Can you work these out from the model? Positions are in its coordinate system, mm. A direction names the side the tool comes from. Coordinates: 2 decimals unless noted, no trailing zeros. Order: outer loops, then holes, each group sorted by start corner. A loop starts at its lowest first (then second) coordinate and runs counter-clockwise, first axis right, second up. Notation, with made-up numbers: (69.5, 7) -> (80.5, 7) arc R21 cw to (80.5, 16) -> close; hole circle Ø11 at (-26, 87.25). An arc over 180 degrees is marked (long way). Write item = value, one per line.
```python
from build123d import *

# Parameters (mm, degrees)
F0_W     = 19.506821
F0_H     = 90
F1_DEPTH = 9


with BuildPart() as f1:
    # F0 (on Front) → F1 (new body)
    with BuildSketch(Plane.XZ):
        with BuildLine():
            Line((100.506821, -115.94898), (100.506821, -102.44898))
            Line((100.506821, -102.44898), (81, -102.44898))
            Line((81, -102.44898), (81, -112.44898))
            ThreePointArc((81, -112.44898), (79.535534, -115.984513), (76, -117.44898))
            Line((76, -117.44898), (-76, -117.44898))
            ThreePointArc((-76, -117.44898), (-79.535534, -115.984513), (-81, -112.44898))
            Line((-81, -112.44898), (-81, -102.44898))
            Line((-81, -102.44898), (-101, -102.44898))
            Line((-101, -102.44898), (-101, -115.94898))
            ThreePointArc((-101, -115.94898), (-99.93934, -116.388319), (-99.5, -117.44898))
            ThreePointArc((-99.5, -117.44898), (-101, -118.94898), (-102.5, -117.44898))
            Line((-102.5, -117.44898), (-110, -117.44898))
            Line((-110, -117.44898), (-110, -122.44898))
            ThreePointArc((-110, -122.44898), (-104.142136, -136.591115), (-90, -142.44898))
            Line((-90, -142.44898), (90, -142.44898))
            ThreePointArc((90, -142.44898), (104.142136, -136.591115), (110, -122.44898))
            Line((110, -122.44898), (110, -117.44898))
            Line((110, -117.44898), (102.006821, -117.44898))
            ThreePointArc((102.006821, -117.44898), (99.446161, -118.50964), (100.506821, -115.94898))
        make_face()
        with Locations((90.753411, -57.44898)):
            Rectangle(F0_W, F0_H)
        with BuildLine():
            Line((90, 137.55102), (-90, 137.55102))
            ThreePointArc((-90, 137.55102), (-104.142136, 131.693156), (-110, 117.55102))
            Line((-110, 117.55102), (-110, 112.55102))
            Line((-110, 112.55102), (-102.5, 112.55102))
            ThreePointArc((-102.5, 112.55102), (-101, 114.05102), (-99.5, 112.55102))
            ThreePointArc((-99.5, 112.55102), (-99.93934, 111.49036), (-101, 111.05102))
            Line((-101, 111.05102), (-101, -12.44898))
            Line((-101, -12.44898), (-81, -12.44898))
            Line((-81, -12.44898), (-81, -7.44898))
            ThreePointArc((-81, -7.44898), (-79.535534, -3.913446), (-76, -2.44898))
            Line((-76, -2.44898), (-61, -2.44898))
            Line((-61, -2.44898), (-61, 17.55102))
            Line((-61, 17.55102), (-76, 17.55102))
            ThreePointArc((-76, 17.55102), (-79.535534, 19.015487), (-81, 22.55102))
            Line((-81, 22.55102), (-81, 107.55102))
            ThreePointArc((-81, 107.55102), (-79.535534, 111.086554), (-76, 112.55102))
            Line((-76, 112.55102), (76, 112.55102))
            ThreePointArc((76, 112.55102), (79.535534, 111.086554), (81, 107.55102))
            Line((81, 107.55102), (81, 22.55102))
            ThreePointArc((81, 22.55102), (79.535534, 19.015487), (76, 17.55102))
            Line((76, 17.55102), (60.506821, 17.55102))
            Line((60.506821, 17.55102), (60.506821, -2.44898))
            Line((60.506821, -2.44898), (76, -2.44898))
            ThreePointArc((76, -2.44898), (79.535534, -3.913446), (81, -7.44898))
            Line((81, -7.44898), (81, -12.44898))
            Line((81, -12.44898), (100.506821, -12.44898))
            Line((100.506821, -12.44898), (100.506821, 111.05102))
            ThreePointArc((100.506821, 111.05102), (99.446161, 113.611681), (102.006821, 112.55102))
            Line((102.006821, 112.55102), (110, 112.55102))
            Line((110, 112.55102), (110, 117.55102))
            ThreePointArc((110, 117.55102), (104.142136, 131.693156), (90, 137.55102))
        make_face()
    extrude(amount=-F1_DEPTH)


solid = f1.part
```
Item 1: If I drill on probe 1 along Z at (x, y) = (-64, 0.75); probe 2 along Z at (x, y) = (33, 7.5); probe 3 along X at (y, z) = (7.25, 2.5), over which ranges is the centre line in solid material (lowest first)?
A:
probe_1 = -142.45 to -117.45, -2.45 to 17.55, 112.55 to 137.55
probe_2 = -142.45 to -117.45, 112.55 to 137.55
probe_3 = -101 to -61, 60.51 to 100.51
Item 2: I want a section at A-A, the plane z = 88.5. Please give me the cut outline in (x, y), plus the area to 3 significant figures.
A:
outline = (-101, 0) -> (-81, 0) -> (-81, 9) -> (-101, 9) -> close; (81, 0) -> (100.51, 0) -> (100.51, 9) -> (81, 9) -> close
area = 356 mm2
Item 3: For faces 4 (the flat face through (-101, 4, 50)), 5 (the flat face through (106, 4, -117.449)), 6 (the cylindrical face through (104.297, 4.437, 131.537)), 7 (the flat face through (1, 4, 137.551)), 8 (the flat face through (-61, 4, 7)), which set-ups out of +Z, -Z, +X, -X, +Y, -Y let a thin tool reach every point of the face, with its end or its side?
A:
face_4 = -X, +Y, -Y
face_5 = +X, +Y, -Y
face_6 = +Z, +X, +Y, -Y
face_7 = +Z, +X, -X, +Y, -Y
face_8 = +Y, -Y
Item 4: I'm going to push flat-ended pins straight in: P1, Ø4.5, axis at y = 6, z = -108.5, coming from the -X side; P2, Ø5, axis at y = 2, z = -106.5, coming from the +X side; P3, Ø2, axis at x = -105, y = 6, coming from the +Z side. Where does each tip first touch, or does it pass through?
A:
P1 = -101
P2 = 100.51
P3 = 131.83
Item 5: If we mould it in two halves opening along X, with no side actions, what happens to faces 1 (the flat face through (-101, 4, -109)), 2 (the flat face through (-91, 4, -102.449)), 3 (the flat face through (1, 4, -117.449))? For each: pulls with the +X half, pulls with the -X half, needs draft (parallel to the pull), parting line crosses it, or undercut.
A:
face_1 = pulls with the -X half
face_2 = needs draft
face_3 = undercut
